Here's how the part is built. I have some questions about the finished solid (model axes, mm). Face numbers are marked on the shaded views. A direction names the side the tool comes from. Coordinates: 2 decimals unless noted, no trailing zeros. Loops run counter-clockwise (first coordinate to the right, second up) from the corner with the lowest first, then second, coordinate; pieces in that order, holes last.
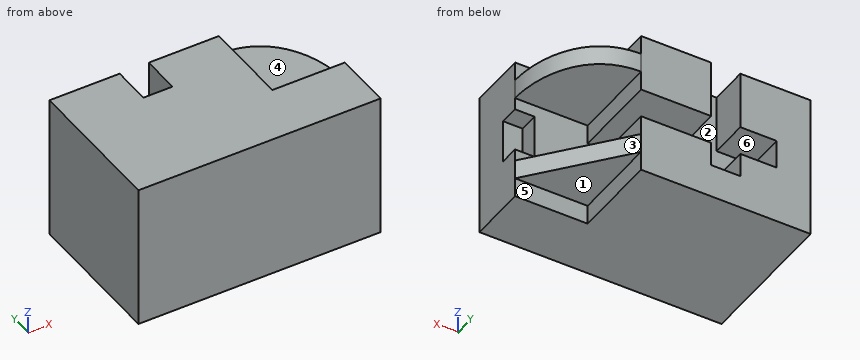
```python
from build123d import *

# Parameters (mm, degrees)
SKETCH_1_W          = 50
SKETCH_1_H          = 30
EXTRUDE_1_DEPTH     = 30
SKETCH_2_W          = 15
SKETCH_2_H          = 18
CUT_EXTRUDE_1_DEPTH = 42.833001327
SKETCH_3_W          = 14.5
SKETCH_3_H          = 6
CUT_EXTRUDE_2_DEPTH = 18
SKETCH_3_3_W        = 6
SKETCH_3_3_H        = 12
SKETCH_3_3_H_2      = 6
SKETCH_3_3_H_3      = 5
SKETCH_3_3_W_2      = 7.5
CUT_EXTRUDE_3_DEPTH = 8
RIB_START           = -2
RIB_1_DEPTH         = 4
RIB_2_REACH         = 39.762
SKETCH_5_WALL_W     = 100.955579594
SKETCH_5_WALL_H     = 4
SKETCH_6_W          = 4
SKETCH_6_H          = 9
CUT_EXTRUDE_4_DEPTH = 4


# Read off the part's stored shape, not the designer's step: Ребро1
with BuildPart() as part:
    # Эскиз1 → Бобышка-Вытянуть1 (new body)
    with BuildSketch(Plane.XY):
        Rectangle(SKETCH_1_W, SKETCH_1_H)
    extrude(amount=EXTRUDE_1_DEPTH)

    # Эскиз2 → Вырез-Вытянуть1 (cut, through all)
    with BuildSketch(Plane.XY.offset(30)):
        with Locations((17.5, 6)):
            Rectangle(SKETCH_2_W, SKETCH_2_H)
    extrude(amount=-CUT_EXTRUDE_1_DEPTH, mode=Mode.SUBTRACT)

    # Эскиз3 → Вырез-Вытянуть2 (cut)
    with BuildSketch(Plane(origin=(0, 15, 0), x_dir=(1, 0, 0), z_dir=(0, 1, 0))):
        with Locations((2.75, -15)):
            Rectangle(SKETCH_3_W, SKETCH_3_H)
    extrude(amount=-CUT_EXTRUDE_2_DEPTH, mode=Mode.SUBTRACT)

    # Эскиз3<3> → Вырез-Вытянуть3 (cut)
    with BuildSketch(Plane(origin=(0, 15, 0), x_dir=(1, 0, 0), z_dir=(0, 1, 0))):
        with Locations((-7.5, -24)):
            Rectangle(SKETCH_3_3_W, SKETCH_3_3_H)
        with Locations((-7.5, -15)):
            Rectangle(SKETCH_3_3_W, SKETCH_3_3_H_2)
        with Locations((-7.5, -9.5)):
            Rectangle(SKETCH_3_3_W, SKETCH_3_3_H_3)
        with Locations((-14.25, -15)):
            Rectangle(SKETCH_3_3_W_2, SKETCH_3_3_H_2)
    extrude(amount=-CUT_EXTRUDE_3_DEPTH, mode=Mode.SUBTRACT)

    # Ребро1 outline → Ребро1 (add)
    with BuildSketch(Plane.XY.offset(24).offset(RIB_START)):
        with BuildLine():
            add(Edge.make_bspline(
                [(10, 15), (20.842232601, 15), (25, 4.810249676), (25, -3)],
                knots=[0, 0, 0, 0, 1, 1, 1, 1], degree=3))
            Line((10, 15), (10, -3))
            Line((10, -3), (25, -3))
        make_face()
    extrude(amount=RIB_1_DEPTH)

    # Эскиз5 wall → Ребро2 (add, up to next)
    with BuildSketch(Plane(origin=(17.5, 6, 6), x_dir=(-0.640184399664, 0.768221279597, 0), z_dir=(-0.768221279597, -0.640184399664, 0)), mode=Mode.PRIVATE) as rib_2_sk1:
        Rectangle(SKETCH_5_WALL_W, SKETCH_5_WALL_H)
    rib_2_tool1 = extrude(rib_2_sk1.sketch, amount=RIB_2_REACH, mode=Mode.PRIVATE) - part.part
    add(rib_2_tool1.solids().sort_by_distance((17.5, 6, 6))[0])

    # Эскиз6 → Вырез-Вытянуть4 (cut)
    with BuildSketch(Plane(origin=(0, -3, 0), x_dir=(1, 0, 0), z_dir=(0, 1, 0))):
        with Locations((23, -15)):
            Rectangle(SKETCH_6_W, SKETCH_6_H)
    extrude(amount=-CUT_EXTRUDE_4_DEPTH, mode=Mode.SUBTRACT)


solid = part.part
```
1. I want a section at D-D (x = 3). Please give me the cut outline in (y, z), then the cut area to 3 significant figures.
2. I want a section at C-C (z = 15.5). Please give me the cut outline in (x, y).
3. We'd pull the mould along X, two halves only. Please class the marked faces 1, 2 and 3: +X half, -X half, draft (parallel to the pull), parting line (faces both ways), or undercut.
4. For pin 1 (1.2 mm diameter, centred on x = 24, z = 17, fed in from +Y); pin 2 (6.5 mm diameter, centred on y = 10, z = 15.5, fed in from +X); pin 3 (4.5 mm diameter, centred on x = 17, y = 7, fed in from +Z), each with a flat end and sliding along its axis, tell me the tip position at first contact or that it passes through.
5. I need wall thicknesses on line 1 along Z through (x, y) = (-11, 12); line 2 along X through (y, z) = (13.5, 28.75); line 3 along Y through (x, z) = (18.5, 20). Which ranges of each line are inside material? Lowest first, please.
6. I want a section at B-B (x = -16). Please give me the cut outline in (y, z).
7. On a 3-axis mill with a long thin cutter (end or side, diameter ignored), from which of +Z, -Z, +X, -X, +Y, -Y can I reach the whole of each face in a straight line? I mean the marked faces 4, 5 and 6. Say none if no direction works.
8. I want a section at A-A (z = 5). Please give me the cut outline in (x, y), then the cut area to 4 significant figures.
Response values:
1. outline: (-15, 0) - (15, 0) - (15, 12) - (-3, 12) - (-3, 18) - (15, 18) - (15, 30) - (-15, 30) - close
1. area: 792 mm2
2. outline: (-25, -15) - (25, -15) - (25, -7) - (21, -7) - (21, -3) - (-4.5, -3) - (-4.5, 7) - (-18, 7) - (-18, 15) - (-25, 15) - close
3. face 1: draft
3. face 2: undercut
3. face 3: +X half
4. pin 1: stops at y = -7
4. pin 2: stops at x = 10
4. pin 3: stops at z = 26
5. line 1: z = 0 to 12, 18 to 30
5. line 2: x = -25 to -10.5, -4.5 to 10
5. line 3: y = -15 to -3
6. outline: (-15, 0) - (15, 0) - (15, 12) - (7, 12) - (7, 18) - (15, 18) - (15, 30) - (-15, 30) - close
7. face 4: +Z, +X, +Y
7. face 5: -Z, +X, +Y
7. face 6: +X, +Y
8. outline: (-25, -15) - (25, -15) - (25, -3) - (10, 15) - (-25, 15) - close
8. area: 1,365 mm2
